from build123d import *

# Parameters (mm, degrees)
ESQUISSE1_R             = 4.15
ESQUISSE1_R_2           = 1.625
BOSS_EXTRU_1_DEPTH      = 2
SALIENTE_EXTRUIR1_START = -1.5
CROQUIS1_R              = 4.15
SALIENTE_EXTRUIR1_DEPTH = 1.5


with BuildPart() as part:
    # Esquisse1 → Boss.-Extru.1 (new body)
    with BuildSketch(Plane.XY):
        with BuildLine():
            Line((3.25, 0), (3.991824339, -2.629250822))
            ThreePointArc((3.991824339, -2.629250822), (6.145300464, -5.784114596), (9.766384215, -7))
            Line((9.766384215, -7), (11.733615785, -7))
            ThreePointArc((11.733615785, -7), (15.354699536, -5.784114596), (17.508175661, -2.629250822))
            Line((17.508175661, -2.629250822), (18.25, 0))
            Line((18.25, 0), (21.5, 0))
            Line((21.5, 0), (21.5, 21.5))
            ThreePointArc((21.5, 21.5), (19.156854249, 27.156854249), (13.5, 29.5))
            Line((13.5, 29.5), (8, 29.5))
            ThreePointArc((8, 29.5), (2.343145751, 27.156854249), (0, 21.5))
            Line((0, 21.5), (0, 0))
            Line((0, 0), (3.25, 0))
        make_face()
        with Locations((10.75, 21.5)):
            Circle(ESQUISSE1_R, mode=Mode.SUBTRACT)
        with Locations((10.75, -1.5)):
            Circle(ESQUISSE1_R_2, mode=Mode.SUBTRACT)
    extrude(amount=BOSS_EXTRU_1_DEPTH)

    # Croquis1 → Saliente-Extruir1 (add)
    with BuildSketch(Plane.XY.offset(SALIENTE_EXTRUIR1_START)):
        with BuildLine():
            ThreePointArc((0, 21.5), (3.148602144, 13.898602061), (10.750000117, 10.75))
            ThreePointArc((10.750000117, 10.75), (18.351397939, 13.898602144), (21.5, 21.5))
            ThreePointArc((21.5, 21.5), (19.156854249, 27.156854249), (13.5, 29.5))
            Line((13.5, 29.5), (8, 29.5))
            ThreePointArc((8, 29.5), (2.343145751, 27.156854249), (0, 21.5))
        make_face()
        with Locations((10.75, 21.5)):
            Circle(CROQUIS1_R, mode=Mode.SUBTRACT)
    saliente_extruir1 = extrude(amount=SALIENTE_EXTRUIR1_DEPTH)

    # Simetría1: Saliente-Extruir1 across plane
    add(saliente_extruir1.mirror(Plane(origin=(0, 0, 1), x_dir=(1, 0, 0), z_dir=(0, 0, -1))))


solid = part.part
Could you check a few things on this model? Use its own coordinates, in mm. A direction names the side the tool comes from. Round coordinates to 2 decimals unless told otherwise and drop trailing zeros. Order: outer loops, then holes, each group sorted by start corner. A loop starts at its lowest first (then second) coordinate and runs counter-clockwise, first axis right, second up.
Q1. Please list where these lines run through material, in increasing order: probe 1 along Y at (x, z) = (10.75, 1.05) (3 decimals); probe 2 along Y at (x, z) = (12.75, -0.65); probe 3 along Z at (x, y) = (5, 5.5).
Geometry says:
probe 1: y = -7 to -3.125, 0.125 to 17.35, 25.65 to 29.5
probe 2: y = 10.94 to 17.86, 25.14 to 29.5
probe 3: z = 0 to 2
Q2. Thinking about a two-plate mould opening in Y: for faces 4 (the face through (9.127, -1.429, 0.986)), 5 (the face through (11, 4, 2)), 6 (the face through (6.1, -5.75, 0.99)), which applies, released by +Y, released by -Y, zero draft, split by the parting line, or undercut?
Geometry says:
face 4: undercut
face 5: zero draft
face 6: released by -Y
Q3. Imagine slicing it at A-A, the plane z = 1.35. List the corners of the cut face in (x, y) for me (3 decimals), then the cut area to 3 significant figures.
Geometry says:
outline: (0, 0) - (3.25, 0) - (3.992, -2.629) arc R6 ccw to (9.766, -7) - (11.734, -7) arc R6 ccw to (17.508, -2.629) - (18.25, 0) - (21.5, 0) - (21.5, 21.5) arc R8 ccw to (13.5, 29.5) - (8, 29.5) arc R8 ccw to (0, 21.5) - close; hole circle Ø8.3 at (10.75, 21.5); hole circle Ø3.25 at (10.75, -1.5)
area: 628 mm2
Q4. Imagine slicing it at B-B, the plane x = 14. List the corners of the cut face in (y, z) for me.
Geometry says:
outline: (-6.56, 0) - (11.25, 0) - (11.25, -1.5) - (18.92, -1.5) - (18.92, 3.5) - (11.25, 3.5) - (11.25, 2) - (-6.56, 2) - close; (24.08, -1.5) - (29.48, -1.5) - (29.48, 3.5) - (24.08, 3.5) - close
Q5. Imagine slicing it at D-D, the plane z = -0.4. List the corners of the cut face in (x, y) for me.
Geometry says:
outline: (0, 21.5) arc R10.75 ccw to (21.5, 21.5) arc R8 ccw to (13.5, 29.5) - (8, 29.5) arc R8 ccw to start; hole circle Ø8.3 at (10.75, 21.5)
Q6. Imagine slicing it at C-C, the plane y = -1.5. List the corners of the cut face in (x, z) for me (3 decimals).
Geometry says:
outline: (3.673, 0) - (9.125, 0) - (9.125, 2) - (3.673, 2) - close; (12.375, 0) - (17.827, 0) - (17.827, 2) - (12.375, 2) - close
Q7. I'm going to push flat-ended pins straight in: P1, Ø0.6, axis at x = 2, z = 1.5, coming from the -Y side; P2, Ø3, axis at x = 14, y = -2.5, coming from the -Z side; P3, Ø3, axis at x = 10.75, y = -1.5, coming from the +Z side; P4, Ø4, axis at x = 11.5, y = 7.5, coming from the +Z side. Where does each tip first touch, or does it pass through?
Geometry says:
P1: stops at y = 0
P2: stops at z = 0
P3: passes through
P4: stops at z = 2
Q8. Which directions (+Z, -Z, +X, -X, +Y, -Y) give clear straight access to the entire face, cutting with the end or side of a thin tool? Please do faces 1 (the face through (20, 0, 1)), 2 (the face through (2, 0, 1)), 3 (the face through (8, 18, -1.5)).
Geometry says:
face 1: +Z, -Z, +X, -Y
face 2: +Z, -Z, -X, -Y
face 3: -Z, +X, -X, +Y, -Y
